Design review of the part built by this model. Coordinates are the model's own, in mm. Face numbers are marked on the shaded views. A direction names the side the tool comes from. Coordinates: 2 decimals unless noted, no trailing zeros. Order: outer loops, then holes, each group sorted by start corner. A loop starts at its lowest first (then second) coordinate and runs counter-clockwise, first axis right, second up.
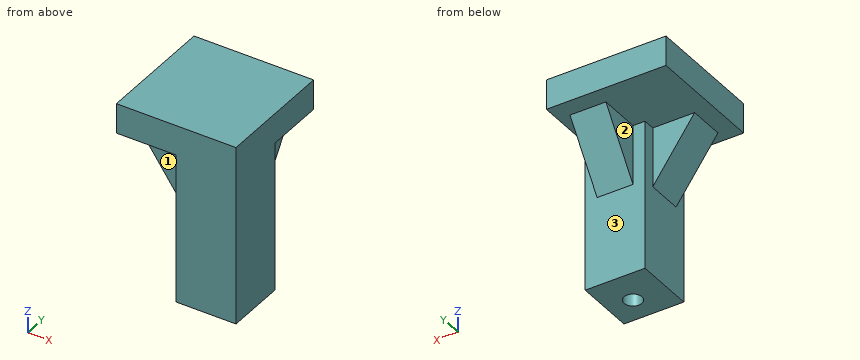
from build123d import *

# Parameters (mm, degrees)
SKETCH_1_W          = 10
SKETCH_1_H          = 10
EXTRUDE_1_DEPTH     = 25
SKETCH_2_R          = 1.5
CUT_EXTRUDE_1_DEPTH = 15
SKETCH_3_W          = 20
SKETCH_3_H          = 20
EXTRUDE_2_DEPTH     = 5
SKETCH_4_W          = 7
SKETCH_4_H          = 3
SKETCH_4_W_2        = 3
SKETCH_4_H_2        = 7
EXTRUDE_3_DEPTH     = 10
CUT_EXTRUDE_2_DEPTH = 10
CUT_EXTRUDE_3_DEPTH = 10


with BuildPart() as part:
    # 草图1 → 凸台-拉伸1 (new body)
    with BuildSketch(Plane.XY):
        with Locations((5, 5)):
            Rectangle(SKETCH_1_W, SKETCH_1_H)
    extrude(amount=EXTRUDE_1_DEPTH)

    # 草图2 → 切除-拉伸1 (cut)
    with BuildSketch(Plane(origin=(0, 0, 0), x_dir=(-1, 0, 0), z_dir=(0, 0, -1))):
        with Locations((-5.707106781, 4.292893219)):
            Circle(SKETCH_2_R)
    extrude(amount=-CUT_EXTRUDE_1_DEPTH, mode=Mode.SUBTRACT)

    # 草图3 → 凸台-拉伸2 (add)
    with BuildSketch(Plane.XY.offset(25)):
        with Locations((0, 10)):
            Rectangle(SKETCH_3_W, SKETCH_3_H)
    extrude(amount=EXTRUDE_2_DEPTH)

    # 草图4 → 凸台-拉伸3 (add)
    with BuildSketch(Plane(origin=(0, 0, 25), x_dir=(-1, 0, 0), z_dir=(0, 0, -1))):
        with Locations((3.5, 6.5)):
            Rectangle(SKETCH_4_W, SKETCH_4_H)
        with Locations((3.5, 3.5)):
            Rectangle(SKETCH_4_W, SKETCH_4_H)
        with Locations((-3.5, 13.5)):
            Rectangle(SKETCH_4_W_2, SKETCH_4_H_2)
        with Locations((-6.5, 13.5)):
            Rectangle(SKETCH_4_W_2, SKETCH_4_H_2)
    extrude(amount=EXTRUDE_3_DEPTH)

    # 草图5 → 切除-拉伸2 (cut)
    with BuildSketch(Plane(origin=(0, 8, 0), x_dir=(1, 0, 0), z_dir=(0, 1, 0))):
        Polygon((-7, -25), (0, -15), (-7, -15), align=None)
    extrude(amount=-CUT_EXTRUDE_2_DEPTH, mode=Mode.SUBTRACT)

    # 草图6 → 切除-拉伸3 (cut)
    with BuildSketch(Plane.ZY.offset(-2)):
        Polygon((15, 10), (25, 17), (15, 17), align=None)
    extrude(amount=-CUT_EXTRUDE_3_DEPTH, mode=Mode.SUBTRACT)


solid = part.part
1. Insertion check: pin 1 (2 mm diameter, centred on y = 13, z = 19.5, fed in from +X); pin 2 (3 mm diameter, centred on y = 7, z = 14, fed in from -X); pin 3 (2 mm diameter, centred on y = 8, z = 9.5, fed in from -X). Each pin has a flat end and moves straight along its axis. Give the tip position at first contact, or say it passes through.
2. For the marked faces 1, 2 and 3, list the 3-axis set-ups (+Z, -Z, +X, -X, +Y, -Y) from which the entire face can be reached by the end or side of a thin tool; tool diameter is ignored.
3. Add section D-D (z = 22.75). Give the boundary of the cut face in (x, y) (3 decimals), and give its area (3 significant figures).
4. To check wall thickness, follow line 1 (Y direction, x = 1.25, z = 12.5); line 2 (Z direction, x = -6, y = 9.25). State the ranges of each line that lie inside material, in increasing order.
5. Add section B-B (z = 7.75). Give the boundary of the cut face in (x, y), and give its area (3 significant figures).
6. Add section A-A (x = 8.75). Give the boundary of the cut face in (y, z), and give its area (3 significant figures).
7. Add section C-C (y = 11.25). Give the boundary of the cut face in (x, z), and give its area (3 significant figures).
Solution:
1. pin 1: stops at x = 8
1. pin 2: stops at x = -0.35
1. pin 3: stops at x = 0
2. face 1: -Z, -X, -Y
2. face 2: -Z, -X, +Y
2. face 3: -Z, +Y
3. outline: (-5.425, 2) - (0, 2) - (0, 0) - (10, 0) - (10, 10) - (8, 10) - (8, 15.425) - (2, 15.425) - (2, 10) - (0, 10) - (0, 8) - (-5.425, 8) - close
3. area: 165 mm2
4. line 1: y = 0 to 10
4. line 2: z = 25 to 30
5. outline: (0, 0) - (10, 0) - (10, 10) - (0, 10) - close; hole circle Ø3 at (5.71, 4.29)
5. area: 92.9 mm2
6. outline: (0, 0) - (10, 0) - (10, 25) - (20, 25) - (20, 30) - (0, 30) - close
6. area: 350 mm2
7. outline: (-10, 25) - (2, 25) - (2, 16.79) - (8, 16.79) - (8, 25) - (10, 25) - (10, 30) - (-10, 30) - close
7. area: 149 mm2
